from build123d import *

# Parameters (mm, degrees)
SKETCH2_R           = 2.5
BOSS_EXTRUDE1_DEPTH = 6.35


with BuildPart() as part:
    # Sketch2 → Boss-Extrude1 (new body)
    with BuildSketch(Plane(origin=(0, 0, 0), x_dir=(1, 0, 0), z_dir=(0, 1, 0))):
        with BuildLine():
            Line((50, 31.8), (50, 81.8))
            ThreePointArc((50, 81.8), (14.644660941, 67.155339059), (0, 31.8))
            Line((0, 31.8), (0, 0))
            Line((0, 0), (50, 0))
            Line((50, 0), (50, 31.8))
        make_face()
        with Locations(Location((45, 31.8, 0), (0, 0, 270))):
            Circle(SKETCH2_R, mode=Mode.SUBTRACT)
        with Locations(Location((6.6, 31.8, 0), (0, 0, 270))):
            Circle(SKETCH2_R, mode=Mode.SUBTRACT)
        with Locations(Location((17.847099602, 58.952900398, 0), (0, 0, 270))):
            Circle(SKETCH2_R, mode=Mode.SUBTRACT)
        with Locations(Location((45, 70.2, 0), (0, 0, 270))):
            Circle(SKETCH2_R, mode=Mode.SUBTRACT)
        with Locations(Location((6.6, 11.8, 0), (0, 0, 270))):
            Circle(SKETCH2_R, mode=Mode.SUBTRACT)
        with Locations(Location((45, 11.8, 0), (0, 0, 270))):
            Circle(SKETCH2_R, mode=Mode.SUBTRACT)
    extrude(amount=BOSS_EXTRUDE1_DEPTH)


solid = part.part
Model file for the job. Use its own axes, mm. Give positions to 0.01 mm unless a question says otherwise; leave off trailing zeros. Order: outer loops, then holes, each group sorted by start corner. A loop starts at its lowest first (then second) coordinate and runs counter-clockwise, first axis right, second up. Notation, with made-up numbers: (40.5, -27) -> (96.5, -27) arc R15 cw to (96.5, -21) -> close; hole circle Ø4 at (-38, 57). An arc over 180 degrees is marked (long way). Use CSV: the item, a comma, the result in double quotes.
1. Drill centre lines: line 1 along X through (y, z) = (5, -31.8); line 2 along Z through (x, y) = (7.5, 2.25); line 3 along X through (y, z) = (4, -11). Where is each one in solid material? Low to high. Write a range as from..to.
Outcome:
line 1,"0..4.1, 9.1..42.5, 47.5..50"
line 2,"-58.14..-34.13, -29.47..-14.13, -9.47..0"
line 3,"0..4.23, 8.97..42.63, 47.37..50"
2. Band-saw the part on A-A, the plane z = -11.8. Give the cut face in (x, y).
Outcome:
outline,"(0, 0) -> (4.1, 0) -> (4.1, 6.35) -> (0, 6.35) -> close; (9.1, 0) -> (42.5, 0) -> (42.5, 6.35) -> (9.1, 6.35) -> close; (47.5, 0) -> (50, 0) -> (50, 6.35) -> (47.5, 6.35) -> close"
3. Band-saw the part on C-C, the plane z = -70.2. Give the cut face in (x, y), then the cut area to 3 significant figures.
Outcome:
outline,"(17.98, 0) -> (42.5, 0) -> (42.5, 6.35) -> (17.98, 6.35) -> close; (47.5, 0) -> (50, 0) -> (50, 6.35) -> (47.5, 6.35) -> close"
area,"172 mm²"
4. Drop flat-ended pins along their axis: pin 1 (3 mm diameter, centred on x = 43, y = 2.5, fed in from -Z); pin 2 (4.5 mm diameter, centred on x = 17.85, z = -58.95, fed in from -Y); pin 3 (3 mm diameter, centred on x = 24.5, y = 1, fed in from -Z). Give the stop position or say it passes through.
Outcome:
pin 1,"z = -81.5"
pin 2,"through"
pin 3,"z = -75.66"
5. Mould opens along X. For faces 1 (the cylindrical face through (45.1, 3.1, -34.3)), 2 (the flat face through (25, 3, 0)), 3 (the flat face through (50, 3, -40)), 4 (the cylindrical face through (15.036, 3.131, -67.542)) say: +X half, -X half, draft (parallel to the pull), parting line (faces both ways), or undercut.
Outcome:
face 1,"undercut"
face 2,"draft"
face 3,"+X half"
face 4,"-X half"
6. Band-saw the part on B-B, the plane y = 5. Give the cut face in (x, z), then the cut area to 3 significant figures.
Outcome:
outline,"(0, -31.8) arc R50 ccw to (50, -81.8) -> (50, 0) -> (0, 0) -> close; hole circle Ø5 at (6.6, -31.8); hole circle Ø5 at (6.6, -11.8); hole circle Ø5 at (17.85, -58.95); hole circle Ø5 at (45, -70.2); hole circle Ø5 at (45, -31.8); hole circle Ø5 at (45, -11.8)"
area,"3,440 mm²"
7. Band-saw the part on D-D, the plane x = 45. Give the cut face in (y, z).
Outcome:
outline,"(0, -81.55) -> (6.35, -81.55) -> (6.35, -72.7) -> (0, -72.7) -> close; (0, -67.7) -> (6.35, -67.7) -> (6.35, -34.3) -> (0, -34.3) -> close; (0, -29.3) -> (6.35, -29.3) -> (6.35, -14.3) -> (0, -14.3) -> close; (0, -9.3) -> (6.35, -9.3) -> (6.35, 0) -> (0, 0) -> close"
